For this review, take the finished solid that the model builds, in its own axes (mm). Face numbers are marked on the shaded views. A direction names the side the tool comes from. Coordinates: 2 decimals unless noted, no trailing zeros. Write each loop counter-clockwise with the first axis right and the second up, starting at its lowest first coordinate (ties: lowest second). Pieces come first, ordered by that corner, then holes. Notation, with made-up numbers: (37.5, 29) - (48.5, 29) arc R9 ccw to (48.5, 40) - close; hole circle Ø5 at (56, -31). An arc over 180 degrees is marked (long way). Use one line per item in the form item = value. Start each with the question number.
1) We need section D-D (x = -7.25). Give the boundary of the cut face in (y, z).
2) For L1, parallel to Y at x = 0, z = 27.5; L2, parallel to Y at x = 2.5, z = 19.5; L3, parallel to Y at x = -3.5, z = 27, list the stretches that pass through material, from the lowest coordinate up. Write a range as from..to.
3) We need section C-C (z = 18.5). Give the boundary of the cut face in (x, y), plus the area to 3 significant figures.
4) We need section A-A (y = -38.5). Give the boundary of the cut face in (x, z), plus the area to 3 significant figures.
5) Mouldability with a two-part tool opening along Y and no side actions: class the marked faces 5, 6 and 7 as pulls with the +Y half, pulls with the -Y half, needs draft (parallel to the pull), parting line crosses it, or undercut.
6) Insertion check: P1, Ø9.5, axis at x = -3.5, y = 37, coming from the -Z side; P2, Ø8, axis at x = 0, y = 38.5, coming from the +Z side; P3, Ø4, axis at x = 3.5, y = 12, coming from the +Z side; P4, Ø9.5, axis at x = -4.5, z = 12.5, coming from the -Y side. Each pin has a flat end and moves straight along its axis. Give the tip position at first contact, or say it passes through.
7) Tool access review of the marked faces 1, 2, 3 and 4: name each direction out of +Z, -Z, +X, -X, +Y, -Y from which nothing blocks a thin tool from reaching the whole face with its end or side.
8) We need section B-B (x = 0). Give the boundary of the cut face in (y, z).
```python
from build123d import *

# Parameters (mm, degrees)
SKETCH1_W           = 19
SKETCH1_H           = 57
BOSS_EXTRUDE1_DEPTH = 12.5
SKETCH2_W           = 19
SKETCH2_H           = 7.5
BOSS_EXTRUDE2_DEPTH = 20
SKETCH3_W           = 19
SKETCH3_H           = 8.5
BOSS_EXTRUDE3_DEPTH = 20
SKETCH4_W           = 19
SKETCH4_H           = 8.5
BOSS_EXTRUDE4_DEPTH = 20
SKETCH5_R           = 5
CUT_EXTRUDE1_DEPTH  = 20


with BuildPart() as part:
    # Sketch1 → Boss-Extrude1 (new body)
    with BuildSketch(Plane.XY):
        Rectangle(SKETCH1_W, SKETCH1_H)
    extrude(amount=BOSS_EXTRUDE1_DEPTH)

    # Sketch2 → Boss-Extrude2 (add)
    with BuildSketch(Plane.XY.offset(12.5)):
        with Locations((0, -24.75)):
            Rectangle(SKETCH2_W, SKETCH2_H)
        with Locations((0, 24.75)):
            Rectangle(SKETCH2_W, SKETCH2_H)
    extrude(amount=BOSS_EXTRUDE2_DEPTH)

    # Sketch3 → Boss-Extrude3 (add)
    with BuildSketch(Plane.XZ.offset(28.5)):
        with Locations((0, 28.25)):
            Rectangle(SKETCH3_W, SKETCH3_H)
    extrude(amount=BOSS_EXTRUDE3_DEPTH)

    # Sketch4 → Boss-Extrude4 (add)
    with BuildSketch(Plane(origin=(0, 28.5, 0), x_dir=(1, 0, 0), z_dir=(0, 1, 0))):
        with Locations((0, -28.25)):
            Rectangle(SKETCH4_W, SKETCH4_H)
    extrude(amount=BOSS_EXTRUDE4_DEPTH)

    # Sketch5 → Cut-Extrude1 (cut)
    with BuildSketch(Plane(origin=(0, 0, 24), x_dir=(-1, 0, 0), z_dir=(0, 0, -1))):
        with Locations((0, 38.5)):
            Circle(SKETCH5_R)
        with Locations((0, -38.5)):
            Circle(SKETCH5_R)
    extrude(amount=-CUT_EXTRUDE1_DEPTH, mode=Mode.SUBTRACT)


solid = part.part
```
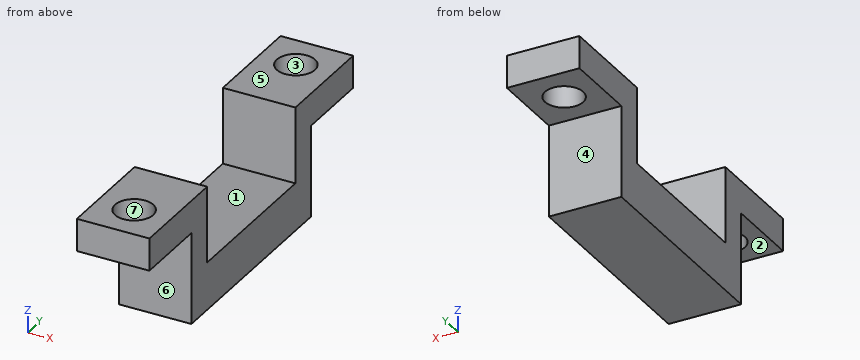
Determined:
q1.outline = (-48.5, 24) - (-28.5, 24) - (-28.5, 0) - (28.5, 0) - (28.5, 24) - (48.5, 24) - (48.5, 32.5) - (21, 32.5) - (21, 12.5) - (-21, 12.5) - (-21, 32.5) - (-48.5, 32.5) - close
q2.L1 = -48.5..-43.5, -33.5..-21, 21..33.5, 43.5..48.5
q2.L2 = -28.5..-21, 21..28.5
q2.L3 = -48.5..-42.07, -34.93..-21, 21..34.93, 42.07..48.5
q3.outline = (-9.5, -28.5) - (9.5, -28.5) - (9.5, -21) - (-9.5, -21) - close; (-9.5, 21) - (9.5, 21) - (9.5, 28.5) - (-9.5, 28.5) - close
q3.area = 285 mm²
q4.outline = (-9.5, 24) - (-5, 24) - (-5, 32.5) - (-9.5, 32.5) - close; (5, 24) - (9.5, 24) - (9.5, 32.5) - (5, 32.5) - close
q4.area = 76.5 mm²
q5.face_5 = needs draft
q5.face_6 = pulls with the -Y half
q5.face_7 = undercut
q6.P1 = 24
q6.P2 = through
q6.P3 = 12.5
q6.P4 = -28.5
q7.face_1 = +Z, +X, -X
q7.face_2 = -Z, +X, -X, -Y
q7.face_3 = +Z, -Z
q7.face_4 = -Z, +X, -X, +Y
q8.outline = (-48.5, 24) - (-43.5, 24) - (-43.5, 32.5) - (-48.5, 32.5) - close; (-33.5, 24) - (-28.5, 24) - (-28.5, 0) - (28.5, 0) - (28.5, 24) - (33.5, 24) - (33.5, 32.5) - (21, 32.5) - (21, 12.5) - (-21, 12.5) - (-21, 32.5) - (-33.5, 32.5) - close; (43.5, 24) - (48.5, 24) - (48.5, 32.5) - (43.5, 32.5) - close
